Verification items for the finished model (mm, model axes). Coordinates: 2 decimals unless noted, no trailing zeros. Loops run counter-clockwise (first coordinate to the right, second up) from the corner with the lowest first, then second, coordinate; pieces in that order, holes last. Notation, with made-up numbers: (75.25, 68.5) -> (110.25, 68.5) arc R23 ccw to (110.25, 85.5) -> close; hole circle Ø7 at (62, 40). An arc over 180 degrees is marked (long way). Write item = value, one per line.
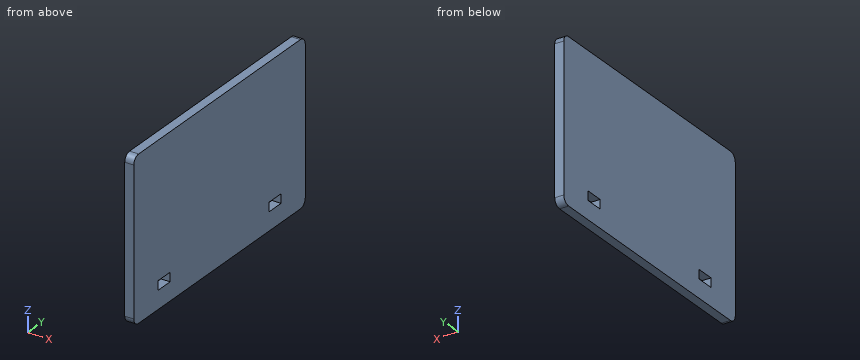
```python
from build123d import *

# Parameters (mm, degrees)
SKETCH1_W           = 55.875
SKETCH1_H           = 90
BOSS_EXTRUDE1_DEPTH = 3.175
SKETCH2_W           = 3.175
SKETCH2_H           = 6.35
CUT_EXTRUDE1_DEPTH  = 54.062081859
FILLET1_R           = 2.54


with BuildPart() as part:
    # Sketch1 → Boss-Extrude1 (new body)
    with BuildSketch(Plane(origin=(0, 0, 0), x_dir=(0, 0, -1), z_dir=(1, 0, 0))):
        Rectangle(SKETCH1_W, SKETCH1_H)
    extrude(amount=BOSS_EXTRUDE1_DEPTH)

    # Sketch2 → Cut-Extrude1 (cut, through all)
    with BuildSketch(Plane(origin=(3.175, 0, 0), x_dir=(0, 0, -1), z_dir=(1, 0, 0))):
        with Locations((20, 29.125)):
            Rectangle(SKETCH2_W, SKETCH2_H)
        with Locations((20, -29.125)):
            Rectangle(SKETCH2_W, SKETCH2_H)
    extrude(amount=-CUT_EXTRUDE1_DEPTH, mode=Mode.SUBTRACT)

    # Fillet1
    fillet1_edges = [part.edges().sort_by_distance(p)[0] for p in [
        (1.5875, 45, 27.9375),
        (1.5875, 45, -27.9375),
        (1.5875, -45, -27.9375),
        (1.5875, -45, 27.9375),
    ]]
    fillet(fillet1_edges, radius=FILLET1_R)


solid = part.part
```
1) Sectioned sample at A-A, the plane y = 30. Record the cut outline in (x, z) (1 decimal).
Ans:
outline = (0, -27.9) -> (3.2, -27.9) -> (3.2, -21.6) -> (0, -21.6) -> close; (0, -18.4) -> (3.2, -18.4) -> (3.2, 27.9) -> (0, 27.9) -> close
2) Material ranges on line 1 (Y direction, x = 1.3, z = -20); line 2 (Z direction, x = 2.25, y = -27); line 3 (Y direction, x = 0.3, z = 26), recorded low to high.
Ans:
line_1 = -45 to -32.3, -25.95 to 25.95, 32.3 to 45
line_2 = -27.94 to -21.59, -18.41 to 27.94
line_3 = -44.93 to 44.93
3) Sectioned sample at B-B, the plane z = -20. Record the cut outline in (x, y) (3 decimals), plus the area to 3 significant figures.
Ans:
outline = (0, -45) -> (3.175, -45) -> (3.175, -32.3) -> (0, -32.3) -> close; (0, -25.95) -> (3.175, -25.95) -> (3.175, 25.95) -> (0, 25.95) -> close; (0, 32.3) -> (3.175, 32.3) -> (3.175, 45) -> (0, 45) -> close
area = 245 mm2
